from build123d import *

# Parameters (mm, degrees)
SKETCH_1_R      = 130
SKETCH_1_R_2    = 1.5
EXTRUDE_2_DEPTH = 3


with BuildPart() as part:
    # 草图1 → 凸台-拉伸2 (new body)
    with BuildSketch(Plane.XY):
        Circle(SKETCH_1_R)
        with Locations((-7, 0)):
            Circle(SKETCH_1_R_2, mode=Mode.SUBTRACT)
        with Locations((0, 7)):
            Circle(SKETCH_1_R_2, mode=Mode.SUBTRACT)
        with Locations((7, 0)):
            Circle(SKETCH_1_R_2, mode=Mode.SUBTRACT)
        with Locations((0, -7)):
            Circle(SKETCH_1_R_2, mode=Mode.SUBTRACT)
        with Locations((-75, -27)):
            Circle(SKETCH_1_R_2, mode=Mode.SUBTRACT)
        with Locations((-75, 27)):
            Circle(SKETCH_1_R_2, mode=Mode.SUBTRACT)
        with Locations((-60.882685902, 51.451905284)):
            Circle(SKETCH_1_R_2, mode=Mode.SUBTRACT)
        with Locations((-14.117314098, 78.451905284)):
            Circle(SKETCH_1_R_2, mode=Mode.SUBTRACT)
        with Locations((14.117314098, 78.451905284)):
            Circle(SKETCH_1_R_2, mode=Mode.SUBTRACT)
        with Locations((60.882685902, 51.451905284)):
            Circle(SKETCH_1_R_2, mode=Mode.SUBTRACT)
        with Locations((75, 27)):
            Circle(SKETCH_1_R_2, mode=Mode.SUBTRACT)
        with Locations((75, -27)):
            Circle(SKETCH_1_R_2, mode=Mode.SUBTRACT)
        with Locations((60.882685902, -51.451905284)):
            Circle(SKETCH_1_R_2, mode=Mode.SUBTRACT)
        with Locations((14.117314098, -78.451905284)):
            Circle(SKETCH_1_R_2, mode=Mode.SUBTRACT)
        with Locations((-14.117314098, -78.451905284)):
            Circle(SKETCH_1_R_2, mode=Mode.SUBTRACT)
        with Locations((-60.882685902, -51.451905284)):
            Circle(SKETCH_1_R_2, mode=Mode.SUBTRACT)
        with BuildLine():
            Line((-14.400742953, 24.012884092), (-18.099614878, 21.87733939))
            ThreePointArc((-18.099614878, 21.87733939), (-25.027817426, 20.725252477), (-31.004889818, 24.413327911))
            Line((-31.004889818, 24.413327911), (-73.035307199, 78.666691732))
            ThreePointArc((-73.035307199, 78.666691732), (-74.94237321, 86.719159796), (-70.130032259, 93.451211287))
            Line((-70.130032259, 93.451211287), (-46.671453646, 106.995027963))
            ThreePointArc((-46.671453646, 106.995027963), (-38.435155561, 107.796611733), (-32.415046659, 102.118810089))
            Line((-32.415046659, 102.118810089), (-6.44546404, 38.592718995))
            ThreePointArc((-6.44546404, 38.592718995), (-6.240033219, 31.572384746), (-10.701871027, 26.148428794))
            Line((-10.701871027, 26.148428794), (-14.400742953, 24.012884092))
        make_face(mode=Mode.SUBTRACT)
        with BuildLine():
            Line((-27.996139118, -0.464967184), (-27.996139118, -4.736056588))
            ThreePointArc((-27.996139118, -4.736056588), (-30.462503858, -11.312099453), (-36.645007071, -14.644358269))
            Line((-36.645007071, -14.644358269), (-104.645007071, -23.917085542))
            ThreePointArc((-104.645007071, -23.917085542), (-112.572181983, -21.542419122), (-115.996139118, -14.008783861))
            Line((-115.996139118, -14.008783861), (-115.996139118, 13.078849492))
            ThreePointArc((-115.996139118, 13.078849492), (-112.572181983, 20.612484753), (-104.645007071, 22.987151173))
            Line((-104.645007071, 22.987151173), (-36.645007071, 13.7144239))
            ThreePointArc((-36.645007071, 13.7144239), (-30.462503858, 10.382165085), (-27.996139118, 3.80612222))
            Line((-27.996139118, 3.80612222), (-27.996139118, -0.464967184))
        make_face(mode=Mode.SUBTRACT)
        with BuildLine():
            Line((13.595396165, 24.477851276), (9.89652424, 26.613395978))
            ThreePointArc((9.89652424, 26.613395978), (5.434686432, 32.03735193), (5.640117252, 39.05768618))
            Line((5.640117252, 39.05768618), (31.609699872, 102.583777273))
            ThreePointArc((31.609699872, 102.583777273), (37.629808773, 108.261578918), (45.866106859, 107.459995148))
            Line((45.866106859, 107.459995148), (69.324685472, 93.916178471))
            ThreePointArc((69.324685472, 93.916178471), (74.137026423, 87.18412698), (72.229960412, 79.131658916))
            Line((72.229960412, 79.131658916), (30.199543031, 24.878295095))
            ThreePointArc((30.199543031, 24.878295095), (24.222470638, 21.190219661), (17.294268091, 22.342306574))
            Line((17.294268091, 22.342306574), (13.595396165, 24.477851276))
        make_face(mode=Mode.SUBTRACT)
        with BuildLine():
            Line((27.996139118, 0.464967184), (27.996139118, 4.736056588))
            ThreePointArc((27.996139118, 4.736056588), (30.462503858, 11.312099453), (36.645007071, 14.644358269))
            Line((36.645007071, 14.644358269), (104.645007071, 23.917085542))
            ThreePointArc((104.645007071, 23.917085542), (112.572181983, 21.542419122), (115.996139118, 14.008783861))
            Line((115.996139118, 14.008783861), (115.996139118, -13.078849492))
            ThreePointArc((115.996139118, -13.078849492), (112.572181983, -20.612484753), (104.645007071, -22.987151173))
            Line((104.645007071, -22.987151173), (36.645007071, -13.7144239))
            ThreePointArc((36.645007071, -13.7144239), (30.462503858, -10.382165085), (27.996139118, -3.80612222))
            Line((27.996139118, -3.80612222), (27.996139118, 0.464967184))
        make_face(mode=Mode.SUBTRACT)
        with BuildLine():
            Line((14.400742953, -24.012884092), (18.099614878, -21.87733939))
            ThreePointArc((18.099614878, -21.87733939), (25.027817426, -20.725252477), (31.004889818, -24.413327911))
            Line((31.004889818, -24.413327911), (73.035307199, -78.666691732))
            ThreePointArc((73.035307199, -78.666691732), (74.94237321, -86.719159796), (70.130032259, -93.451211287))
            Line((70.130032259, -93.451211287), (46.671453646, -106.995027963))
            ThreePointArc((46.671453646, -106.995027963), (38.435155561, -107.796611733), (32.415046659, -102.118810089))
            Line((32.415046659, -102.118810089), (6.44546404, -38.592718995))
            ThreePointArc((6.44546404, -38.592718995), (6.240033219, -31.572384746), (10.701871027, -26.148428794))
            Line((10.701871027, -26.148428794), (14.400742953, -24.012884092))
        make_face(mode=Mode.SUBTRACT)
        with BuildLine():
            Line((-13.595396165, -24.477851276), (-9.89652424, -26.613395978))
            ThreePointArc((-9.89652424, -26.613395978), (-5.434686432, -32.03735193), (-5.640117252, -39.05768618))
            Line((-5.640117252, -39.05768618), (-31.609699872, -102.583777273))
            ThreePointArc((-31.609699872, -102.583777273), (-37.629808773, -108.261578918), (-45.866106859, -107.459995148))
            Line((-45.866106859, -107.459995148), (-69.324685472, -93.916178471))
            ThreePointArc((-69.324685472, -93.916178471), (-74.137026423, -87.18412698), (-72.229960412, -79.131658916))
            Line((-72.229960412, -79.131658916), (-30.199543031, -24.878295095))
            ThreePointArc((-30.199543031, -24.878295095), (-24.222470638, -21.190219661), (-17.294268091, -22.342306574))
            Line((-17.294268091, -22.342306574), (-13.595396165, -24.477851276))
        make_face(mode=Mode.SUBTRACT)
    extrude(amount=EXTRUDE_2_DEPTH)


solid = part.part
CAD build for the part. Positions are in the model's coordinates, mm. Round coordinates to 2 decimals unless told otherwise and drop trailing zeros. Order: outer loops, then holes, each group sorted by start corner. A loop starts at its lowest first (then second) coordinate and runs counter-clockwise, first axis right, second up. Notation, with made-up numbers: (-38, -10.75) - (-3, -10.75) arc R20 ccw to (-3, 8.25) - close; hole circle Ø6 at (22, -33.5). An arc over 180 degrees is marked (long way). Return JSON: item names as keys, results as strings.
(1) Cut at D-D (z = 0.85). State how many separate pieces and enclosed holes the cut face has, then the cut area to 3 significant figures.
Answer key:
{"separate pieces": "1", "enclosed holes": "22", "area": "33,500 mm^2"}
(2) Cut at A-A (x = -111.5). Give the cut face in (y, z).
Answer key:
{"outline": "(-66.84, 0) - (-22.36, 0) - (-22.36, 3) - (-66.84, 3) - close; (21.43, 0) - (66.84, 0) - (66.84, 3) - (21.43, 3) - close"}
(3) Pull direction Y, two halves, no side cores. Call faces 1 (the face through (-51.509, -52.385, 1.479)), 2 (the face through (-2, 2, 0)): +Y half, -Y half, draft (parallel to the pull), parting line (faces both ways), or undercut.
Answer key:
{"face 1": "undercut", "face 2": "draft"}
(4) Pin check, flat tips, straight feed: pin 1 Ø4 at (x, y) = (60.88, 51.45) entering from +Z; pin 2 Ø1.5 at (y, z) = (-2, 2.5) entering from -X; pin 3 Ø1.5 at (y, z) = (-6, 2) entering from +X; pin 4 Ø2.5 at (x, y) = (-14.12, -78.45) entering from +Z. Stop position of each tip, or through.
Answer key:
{"pin 1": "stops at z = 3", "pin 2": "stops at x = -129.99", "pin 3": "stops at x = 129.89", "pin 4": "passes through"}
(5) Cut at C-C (x = 51). Give the cut face in (y, z).
Answer key:
{"outline": "(-119.58, 0) - (-104.5, 0) - (-104.5, 3) - (-119.58, 3) - close; (-50.22, 0) - (-15.67, 0) - (-15.67, 3) - (-50.22, 3) - close; (16.6, 0) - (51.73, 0) - (51.73, 3) - (16.6, 3) - close; (104.5, 0) - (119.58, 0) - (119.58, 3) - (104.5, 3) - close"}
(6) Cut at B-B (y = -45). Give the cut face in (x, z), then the cut area to 3 significant figures.
Answer key:
{"outline": "(-121.96, 0) - (-45.79, 0) - (-45.79, 3) - (-121.96, 3) - close; (-8.07, 0) - (9.06, 0) - (9.06, 3) - (-8.07, 3) - close; (46.95, 0) - (121.96, 0) - (121.96, 3) - (46.95, 3) - close", "area": "505 mm^2"}
(7) Wall check: probe 1 along X at (y, z) = (26.5, 2.25); probe 2 along X at (y, z) = (-96.5, 2.85); probe 3 along X at (y, z) = (-98, 1.55). Give the ranges that are in metal, low to high. Write a range as from..to.
Answer key:
{"probe 1": "x = -127.27..-76.41, -73.59..-32.62, -10.14..10.09, 31.46..73.59, 76.41..127.27", "probe 2": "x = -87.11..-64.85, -29.12..30.12, 64.85..87.11", "probe 3": "x = -85.42..-62.25, -29.74..30.73, 62.25..85.42"}
